Could you check a few things on this model? Use its own coordinates, in mm. A direction names the side the tool comes from. Round coordinates to 2 decimals unless told otherwise and drop trailing zeros. Write each loop counter-clockwise with the first axis right and the second up, starting at its lowest first coordinate (ties: lowest second). Pieces come first, ordered by that corner, then holes. Notation, with made-up numbers: (76, 59.5) -> (96, 59.5) arc R19 ccw to (96, 73.5) -> close; hole circle Ø1 at (-36, -19). An arc over 180 degrees is marked (long way). Answer in a Markdown table with one row per item.
Autodesk Fusion 360 part; units mm, degrees
sketch "Skizze1" plane through (0, 0, 0) normal (0, 0, 1) x (1, 0, 0)
  line L0 (4.5, 4.5) -> (35.5, 4.5)
  line L1 (35.5, 4.5) -> (35.5, 35.5)
  line L2 (35.5, 35.5) -> (4.5, 35.5)
  line L3 (4.5, 35.5) -> (4.5, 4.5)
  line L4 (4.5, 4.5) -> (35.5, 35.5) construction
  line L5 (35.5, 4.5) -> (4.5, 35.5) construction
  circle A0 centre (20, 20) radius 11.5
  circle A1 centre (4.5, 35.5) radius 2
  circle A2 centre (35.5, 35.5) radius 2
  circle A3 centre (4.5, 4.5) radius 2
  circle A4 centre (35.5, 4.5) radius 2
  line L6 (0, 40) -> (40, 40)
  line L7 (40, 40) -> (40, 0)
  line L8 (40, 0) -> (0, 0)
  line L9 (0, 0) -> (0, 40)
  line L10 (0, 40) -> (40, 0) construction
  line L11 (40, 40) -> (0, 0) construction
  point P0 (20, 20)
  point P1 (20, 20)
  dimension "d1" = 31
  dimension "d2" = 31
  dimension "d3" = 23
  dimension "d4" = 4
  dimension "d5" = 4
  dimension "d6" = 4
  dimension "d7" = 4
  dimension "d8" = 40
  dimension "d9" = 40
extrude "Extrusion1" add sketch "Skizze1" along normal blind 10 contours L0 L1 L2 L3 A1 A2 A3 A4 | L6 L7 L8 L9
sketch "Skizze2" plane through (0, 0, 10) normal (0, 0, 1) x (-1, 0, 0)
  circle A0 centre (-4.5, -4.5) radius 2
  circle A1 centre (-35.5, -35.5) radius 2
  circle A2 centre (-35.5, -4.5) radius 2
  circle A3 centre (-20, -20) radius 11.5
  circle A4 centre (-4.5, -35.5) radius 2
  line L0 (0, 0) -> (-40, 0)
  line L1 (-40, 0) -> (-40, -40)
  line L2 (-40, -40) -> (0, -40)
  line L3 (0, -40) -> (0, 0)
  line L4 (0, -31) -> (-40, -31)
  line L5 (-40, -31) -> (-40, -9)
  line L6 (-40, -9) -> (0, -9)
  line L7 (0, -9) -> (0, -31)
  line L8 (0, -31) -> (-40, -9) construction
  line L9 (-40, -31) -> (0, -9) construction
  line L10 (-9, -40) -> (-31, -40)
  line L11 (-31, -40) -> (-31, 0)
  line L12 (-31, 0) -> (-9, 0)
  line L13 (-9, 0) -> (-9, -40)
  line L14 (-9, -40) -> (-31, 0) construction
  line L15 (-31, -40) -> (-9, 0) construction
  point P0 (-20, -20)
  point P1 (-20, -20)
extrude "Extrusion2" add sketch "Skizze2" along normal blind 30 contours A3 L3 L4 L6 L7 L13 | A3 L6 L13 | A3 L4 L13 | A3 L0 L6 L11 L12 L13 | A3 L2 L4 L10 L11 L13 | A3 L6 L11 | A3 L4 L11 | A3 L1 L4 L5 L6 L11
sketch "Skizze3" plane through (0, 0, 40) normal (0, 0, 1) x (-1, 0, 0)
  circle A0 centre (-20, -20) radius 11.5
  line L0 (-9, 0) -> (-31, 0)
  line L1 (-31, 0) -> (-31, -9)
  line L2 (-31, -9) -> (-40, -9)
  line L3 (-40, -9) -> (-40, -31)
  line L4 (-40, -31) -> (-31, -31)
  line L5 (-31, -31) -> (-31, -40)
  line L6 (-31, -40) -> (-9, -40)
  line L7 (-9, -40) -> (-9, -31)
  line L8 (-9, -31) -> (0, -31)
  line L9 (0, -31) -> (0, -9)
  line L10 (0, -9) -> (-9, -9)
  line L11 (-9, -9) -> (-9, 0)
  line L12 (0, -40) -> (-40, -40)
  line L13 (-40, -40) -> (-40, 0)
  line L14 (-40, 0) -> (0, 0)
  line L15 (0, 0) -> (0, -40)
  line L16 (0, -40) -> (-40, 0) construction
  line L17 (-40, -40) -> (0, 0) construction
  point P0 (-20, -20)
extrude "Extrusion3" add sketch "Skizze3" along normal blind 2
extrude "Extrusion4" add 1 faces at (19.7135, 37.1559, 42) along direction (0, 0, 1) blind 13
sketch "Skizze4" plane through (40, 0, 0) normal (1, 0, 0) x (0, 1, 0)
  line L0 (0, 0) -> (40, 0)
  line L1 (40, 0) -> (40, 10)
  line L2 (40, 10) -> (31, 10)
  line L3 (31, 10) -> (31, 40)
  line L4 (31, 40) -> (40, 40)
  line L5 (40, 40) -> (40, 55)
  line L6 (40, 55) -> (0, 55)
  line L7 (0, 55) -> (0, 40)
  line L8 (0, 40) -> (9, 40)
  line L9 (9, 40) -> (9, 10)
  line L10 (9, 10) -> (0, 10)
  line L11 (0, 10) -> (0, 0)
  circle A0 centre (10, 52) radius 2
  circle A1 centre (10, 45) radius 2
  line L12 (10, 52) -> (10, 45)
  dimension "d18" = 4
  dimension "d19" = 4
  dimension "d26" = 7
extrude "Extrusion5" cut sketch "Skizze4" against normal blind 10 contours A0 | A1
fillet "Abrundung1" radius 9 8 edges at (31, 35.5, 40) (35.5, 31, 40) (31, 4.5, 40) (35.5, 9, 40) (4.5, 9, 40) (9, 4.5, 40) (9, 35.5, 40) (4.5, 31, 40)
fillet "Abrundung2" radius 2 1 edges at (30.7218, 15.8414, 55)
1) Imagine slicing it at C-C, the plane y = 35.5. Please give me the cut outline in (x, z), plus the area to 3 significant figures.
Findings:
| item | result |
|---|---|
| outline | (0, 0) -> (2.5, 0) -> (2.5, 10) -> (0, 10) -> close; (0, 38.79) -> (4.5, 38.79) arc R9 cw to (9, 31) -> (9, 10) -> (6.5, 10) -> (6.5, 0) -> (33.5, 0) -> (33.5, 10) -> (31, 10) -> (31, 31) arc R9 cw to (35.5, 38.79) -> (40, 38.79) -> (40, 55) -> (0, 55) -> close; (37.5, 0) -> (40, 0) -> (40, 10) -> (37.5, 10) -> close |
| area | 1,620 mm^2 |
2) For faces 1 (the face through (35, 38, 10)), 2 (the face through (9, 4, 20)), 3 (the face through (33, 5, 10)), 4 (the face through (4, 38, 10)), which set-ups out of +Z, -Z, +X, -X, +Y, -Y let a thin tool reach every point of the face, with its end or its side?
Findings:
| item | result |
|---|---|
| face 1 | +X, +Y |
| face 2 | -X, -Y |
| face 3 | +X, -Y |
| face 4 | -X, +Y |
3) Thinking about a two-plate mould opening in X: for faces 5 (the face through (32.68, 3.44, 36.24)), 6 (the face through (7.32, 36.56, 36.24)), 7 (the face through (4.066, 37.452, 4.93)), 8 (the face through (2.9, 5.7, 4.9)), which applies, +X half, -X half, draft (parallel to the pull), parting line (faces both ways), or undercut?
Findings:
| item | result |
|---|---|
| face 5 | +X half |
| face 6 | -X half |
| face 7 | undercut |
| face 8 | undercut |
4) For pin 1 (4.5 mm diameter, centred on x = 4, z = 23, fed in from -Y); pin 2 (3 mm diameter, centred on y = 34.5, z = 19.5, fed in from +X); pin 3 (2.5 mm diameter, centred on y = 4, z = 16.5, fed in from -X), each with a flat end and sliding along its axis, tell me the tip position at first contact or that it passes through.
Findings:
| item | result |
|---|---|
| pin 1 | stops at y = 9 |
| pin 2 | stops at x = 31 |
| pin 3 | stops at x = 9 |
5) Please list where these lines run through material, in increasing order: line 1 (Y direction, x = 35.5, z = 5); line 2 (Z direction, x = 36, y = 10).
Findings:
| item | result |
|---|---|
| line 1 | y = 0 to 2.5, 6.5 to 33.5, 37.5 to 40 |
| line 2 | z = 0 to 43, 47 to 50, 54 to 55 |
6) Imagine slicing it at A-A, the plane z = 17.5. Please give me the cut outline in (x, y), plus the area to 3 significant figures.
Findings:
| item | result |
|---|---|
| outline | (0, 9) -> (9, 9) -> (9, 0) -> (31, 0) -> (31, 9) -> (40, 9) -> (40, 31) -> (31, 31) -> (31, 40) -> (9, 40) -> (9, 31) -> (0, 31) -> close; hole circle Ø23 at (20, 20) |
| area | 861 mm^2 |
7) Imagine slicing it at B-B, the plane x = 34.5. Please give me the cut outline in (y, z).
Findings:
| item | result |
|---|---|
| outline | (0, 0) -> (2.77, 0) -> (2.77, 10) -> (0, 10) -> close; (0, 38.12) -> (5.5, 38.12) arc R9 cw to (9, 31) -> (9, 10) -> (6.23, 10) -> (6.23, 0) -> (33.77, 0) -> (33.77, 10) -> (31, 10) -> (31, 31) arc R9 cw to (34.5, 38.12) -> (40, 38.12) -> (40, 55) -> (0, 55) -> close; (37.23, 0) -> (40, 0) -> (40, 10) -> (37.23, 10) -> close; hole circle Ø4 at (10, 45); hole circle Ø4 at (10, 52) |
